The model under review builds one solid part; all positions refer to its coordinate system, in mm. A direction names the side the tool comes from. Give positions to 0.01 mm unless a question says otherwise; leave off trailing zeros. Order: outer loops, then holes, each group sorted by start corner. A loop starts at its lowest first (then second) coordinate and runs counter-clockwise, first axis right, second up.
```python
from build123d import *

# Parameters (mm, degrees)
F0_R     = 11.2
F1_DEPTH = 25


# Not quite as in the source:
# - ends of sketch curves that miss each other by under 0.0002 mm in the source are joined


with BuildPart() as f1:
    # F0 (on Top) → F1 (new body)
    with BuildSketch(Plane.XY):
        with BuildLine():
            ThreePointArc((0.2302689957, -13.1979913695), (9.4148699073, -9.2520389444), (13.2, 0))
            ThreePointArc((13.2, 0), (9.3338018159, 9.3338172074), (-2.1767e-05, 13.2))
            ThreePointArc((-2.1767e-05, 13.2), (-13.1994921512, 0.115788384), (-0.2315896221, -13.1979682621))
            Line((-0.2315896221, -13.1979682621), (0.2302689957, -13.1979913695))
        make_face()
        Circle(F0_R, mode=Mode.SUBTRACT)
        with BuildLine():
            ThreePointArc((-2.1767e-05, 13.2), (9.3338018159, 9.3338172074), (13.2, 0))
            ThreePointArc((13.2, 0), (9.4148699073, -9.2520389444), (0.2302689957, -13.1979913695))
            Line((0.2302689957, -13.1979913695), (40.3773476235, -13.1999999835))
            ThreePointArc((40.3773476235, -13.1999999835), (27.1780080417, 0.0003193237), (40.3779862708, 13.2))
            Line((40.3779862708, 13.2), (-2.1767e-05, 13.2))
        make_face()
        with BuildLine():
            ThreePointArc((-0.2315896221, -13.1979682621), (-13.1994921512, 0.115788384), (-2.1767e-05, 13.2))
            Line((-2.1767e-05, 13.2), (-44.8087825295, 13.1998595259))
            ThreePointArc((-44.8087825295, 13.1998595259), (-35.5143647291, 9.3122541296), (-31.6696799576, 0))
            ThreePointArc((-31.6696799576, 0), (-35.4182181161, -9.2146551242), (-44.534811633, -13.1957517105))
            Line((-44.534811633, -13.1957517105), (-0.2315896221, -13.1979682621))
        make_face()
        with BuildLine():
            ThreePointArc((-0.2315896221, -13.1979682621), (-0.0006604143, -13.1999999835), (0.2302689957, -13.1979913695))
            Line((0.2302689957, -13.1979913695), (-0.2315896221, -13.1979682621))
        make_face()
        with BuildLine():
            ThreePointArc((-31.6696799576, 0), (-35.5143647291, 9.3122541296), (-44.8087825295, 13.1998595259))
            ThreePointArc((-44.8087825295, 13.1998595259), (-46.7206749928, 13.0695760214), (-48.593555626, 12.6638363068))
            ThreePointArc((-48.593555626, 12.6638363068), (-52.8729419323, 10.4970375709), (-56.0955079711, 6.9441187643))
            ThreePointArc((-56.0955079711, 6.9441187643), (-56.4810242111, -6.2782708311), (-45.2058686841, -13.1957181366))
            Line((-45.2058686841, -13.1957181366), (-44.534811633, -13.1957517105))
            ThreePointArc((-44.534811633, -13.1957517105), (-35.4182181161, -9.2146551242), (-31.6696799576, 0))
        make_face()
        with Locations((-44.8696799576, 0)):
            Circle(F0_R, mode=Mode.SUBTRACT)
        with BuildLine():
            ThreePointArc((53.5780080378, 0), (49.7118098537, 9.3338172074), (40.3779862708, 13.2))
            ThreePointArc((40.3779862708, 13.2), (27.1780080417, 0.0003193237), (40.3773476235, -13.1999999835))
            ThreePointArc((40.3773476235, -13.1999999835), (44.5067810862, -12.5376725558), (48.2217520277, -10.6167641125))
            ThreePointArc((48.2217520277, -10.6167641125), (52.1631134821, -5.9456950533), (53.5780080378, 0))
        make_face()
        with Locations((40.3780080378, 0)):
            Circle(F0_R, mode=Mode.SUBTRACT)
        with BuildLine():
            ThreePointArc((-45.2058686841, -13.1957181366), (-44.8703403719, -13.1999999835), (-44.534811633, -13.1957517105))
            Line((-44.534811633, -13.1957517105), (-45.2058686841, -13.1957181366))
        make_face()
        with BuildLine():
            ThreePointArc((-56.0955079711, 6.9441187643), (-52.8729419323, 10.4970375709), (-48.593555626, 12.6638363068))
            Line((-48.593555626, 12.6638363068), (-63.987724483, 25.5667958409))
            Line((-63.987724483, 25.5667958409), (-56.0955079711, 6.9441187643))
        make_face()
        with BuildLine():
            Line((62.9060839376, -22.9247582743), (53.5780080378, 0))
            ThreePointArc((53.5780080378, 0), (52.1631134821, -5.9456950533), (48.2217520277, -10.6167641125))
            Line((48.2217520277, -10.6167641125), (62.9060839376, -22.9247582743))
        make_face()
    extrude(amount=F1_DEPTH)


solid = f1.part
```
Item 1: Take a section at B-B (x = 33.5). Give the boundary of the cut face in (y, z).
Values found:
outline: (-13.2, 0) - (-8.84, 0) - (-8.84, 25) - (-13.2, 25) - close; (8.84, 0) - (13.2, 0) - (13.2, 25) - (8.84, 25) - close
Item 2: Draft analysis for pull direction X (two halves, no side actions). For faces 4 (the cylindrical face through (49.814, 9.231, 12.325)), 5 (the flat face through (-60.1, 16.39, 12.32)), 6 (the flat face through (55.461, -16.685, 12.325)), state which applies: released by +X, released by -X, zero draft, split by the parting line, or undercut.
Values found:
face 4: released by +X
face 5: released by -X
face 6: undercut
Item 3: Clearance check with flat-ended pins moving along their axes: pin 1 Ø5 at (x, z) = (11, 4.5) entering from +Y; pin 2 Ø7.5 at (x, z) = (-21.5, 18) entering from -Y; pin 3 Ø1.5 at (x, z) = (-47, 10) entering from +Y. State where each tip first meets the part, or that it passes through.
Values found:
pin 1: stops at y = 13.2
pin 2: stops at y = -13.2
pin 3: stops at y = 13.13
Item 4: Take a section at D-D (y = 4.5). Give the boundary of the cut face in (x, z).
Values found:
outline: (-57.28, 0) - (-55.13, 0) - (-55.13, 25) - (-57.28, 25) - close; (-34.61, 0) - (-10.26, 0) - (-10.26, 25) - (-34.61, 25) - close; (10.26, 0) - (30.12, 0) - (30.12, 25) - (10.26, 25) - close; (50.63, 0) - (52.79, 0) - (52.79, 25) - (50.63, 25) - close
Item 5: For faces 1 (the cylindrical face through (44.451, -12.556, 12.325)), 2 (the flat face through (58.3, -11.6, 12.3)), 3 (the cylindrical face through (-46.694, 13.073, 12.325)), list the 3-axis set-ups (+Z, -Z, +X, -X, +Y, -Y) from which the entire face can be reached by the end or side of a thin tool; tool diameter is ignored.
Values found:
face 1: +Z, -Z, -Y
face 2: +Z, -Z, +X, +Y
face 3: +Z, -Z, +Y
Item 6: Take a section at C-C (z = 1.75). Give the boundary of the cut face in (x, y), and give its area (3 significant figures).
Values found:
outline: (-63.99, 25.57) - (-56.1, 6.94) arc R13.2 ccw to (-44.53, -13.2) - (-0.23, -13.2) arc R13.2 ccw to (0.23, -13.2) - (40.38, -13.2) arc R13.2 ccw to (48.22, -10.62) - (62.91, -22.92) - (53.58, 0) arc R13.2 ccw to (40.38, 13.2) - (0, 13.2) - (-44.81, 13.2) arc R13.2 ccw to (-48.59, 12.66) - close; hole circle Ø22.4 at (-44.87, 0); hole circle Ø22.4 at (0, 0); hole circle Ø22.4 at (40.38, 0)
area: 1,800 mm2
Item 7: For line 1 (Y direction, x = 0, z = 9.25); line 2 (X direction, y = 9.5, z = 20); line 3 (X direction, y = -1, z = 14.75), list the stretches that pass through material, from the lowest coordinate up.
Values found:
line 1: y = -13.2 to -11.2, 11.2 to 13.2
line 2: x = -57.18 to -50.8, -38.94 to -5.93, 5.93 to 34.45, 46.31 to 49.54
line 3: x = -58.03 to -56.02, -33.71 to -11.16, 11.16 to 29.22, 51.53 to 53.98
Item 8: Take a section at A-A (y = -3). Give the boundary of the cut face in (x, z), and give its area (3 significant figures).
Values found:
outline: (-57.72, 0) - (-55.66, 0) - (-55.66, 25) - (-57.72, 25) - close; (-34.08, 0) - (-10.79, 0) - (-10.79, 25) - (-34.08, 25) - close; (10.79, 0) - (29.59, 0) - (29.59, 25) - (10.79, 25) - close; (51.17, 0) - (54.8, 0) - (54.8, 25) - (51.17, 25) - close
area: 1,190 mm2
